from build123d import *

# Parameters (mm, degrees)
SKETCH1_W           = 64.8
SKETCH1_H           = 159
SKETCH1_R           = 1.5
BOSS_EXTRUDE1_DEPTH = 3
SKETCH7_W           = 2.2
SKETCH7_H           = 52
CUT_EXTRUDE4_DEPTH  = 86.901164136
CUT_EXTRUDE6_DEPTH  = 86.901164136
SKETCH12_R          = 1.25
CUT_EXTRUDE8_DEPTH  = 10


with BuildPart() as part:
    # Sketch1 → Boss-Extrude1 (new body)
    with BuildSketch(Plane(origin=(0, 0, 0), x_dir=(1, 0, 0), z_dir=(0, 1, 0))):
        Rectangle(SKETCH1_W, SKETCH1_H)
        with Locations(Location((-27.4, 69.5, 0), (0, 0, 270))):
            Circle(SKETCH1_R, mode=Mode.SUBTRACT)
        with Locations(Location((27.4, 69.5, 0), (0, 0, 270))):
            Circle(SKETCH1_R, mode=Mode.SUBTRACT)
        with Locations(Location((27.4, 31.5, 0), (0, 0, 270))):
            Circle(SKETCH1_R, mode=Mode.SUBTRACT)
        with Locations(Location((-27.4, 31.5, 0), (0, 0, 270))):
            Circle(SKETCH1_R, mode=Mode.SUBTRACT)
    extrude(amount=BOSS_EXTRUDE1_DEPTH)

    # Sketch7 → Cut-Extrude4 (cut, through all)
    with BuildSketch(Plane(origin=(0, 3, 0), x_dir=(1, 0, 0), z_dir=(0, 1, 0))):
        with Locations((-27.6, -8.5)):
            Rectangle(SKETCH7_W, SKETCH7_H)
        with Locations((27.6, -8.5)):
            Rectangle(SKETCH7_W, SKETCH7_H)
        with Locations((-21.9, -8.5)):
            Rectangle(SKETCH7_W, SKETCH7_H)
        with Locations((21.9, -8.5)):
            Rectangle(SKETCH7_W, SKETCH7_H)
    extrude(amount=-CUT_EXTRUDE4_DEPTH, mode=Mode.SUBTRACT)

    # Sketch9 → Cut-Extrude6 (cut, through all)
    with BuildSketch(Plane(origin=(0, 3, 0), x_dir=(1, 0, 0), z_dir=(0, 1, 0))):
        Polygon((-27.4, -65.75), (27.4, -65.75), (27.4, -58.25), (8.75, -58.25), (8.75, -50.25), (-8.75, -50.25), (-8.75, -58.25), (-27.4, -58.25), align=None)
    extrude(amount=-CUT_EXTRUDE6_DEPTH, mode=Mode.SUBTRACT)

    # Sketch12 → Cut-Extrude8 (cut)
    with BuildSketch(Plane(origin=(0, 3, 0), x_dir=(1, 0, 0), z_dir=(0, 1, 0))):
        with Locations(Location((-24.5, -47.5, 0), (0, 0, 270))):
            Circle(SKETCH12_R)
        with Locations(Location((24.5, -47.5, 0), (0, 0, 270))):
            Circle(SKETCH12_R)
        with Locations(Location((24.5, -76.5, 0), (0, 0, 270))):
            Circle(SKETCH12_R)
        with Locations(Location((-24.5, -76.5, 0), (0, 0, 270))):
            Circle(SKETCH12_R)
    extrude(amount=-CUT_EXTRUDE8_DEPTH, mode=Mode.SUBTRACT)


solid = part.part
Work out the finished part from the listing and answer in its coordinate system (mm). A direction names the side the tool comes from. Give positions to 0.01 mm unless a question says otherwise; leave off trailing zeros. Order: outer loops, then holes, each group sorted by start corner. A loop starts at its lowest first (then second) coordinate and runs counter-clockwise, first axis right, second up. Notation, with made-up numbers: M 4.25,-10 L 41.25,-10 A36 ccw 41.25,28 Z; hole C -8,83 d6. An arc over 180 degrees is marked long. Return JSON: item names as keys, results as strings.
Q1. Find section C-C, the plane z = 63. Write down the section's boundary in (x, y).
Answer below:
{"outline": "M -32.4,0 L -27.4,0 L -27.4,3 L -32.4,3 Z; M 27.4,0 L 32.4,0 L 32.4,3 L 27.4,3 Z"}
Q2. Find section B-B, the plane x = -12. Write down the section's boundary in (y, z).
Answer below:
{"outline": "M 0,-79.5 L 3,-79.5 L 3,58.25 L 0,58.25 Z; M 0,65.75 L 3,65.75 L 3,79.5 L 0,79.5 Z"}
Q3. Find the intervals of material crossed by line 1 along X through (y, z) = (2.3, 76.5); line 2 along X through (y, z) = (1.7, -31.5); line 3 along Z through (x, y) = (-22, 1.35), in increasing order. Write a range as [from, to].
Answer below:
{"line 1": "x = [-32.4, -25.75], [-23.25, 23.25], [25.75, 32.4]", "line 2": "x = [-32.4, -28.9], [-25.9, 25.9], [28.9, 32.4]", "line 3": "z = [-79.5, -17.5], [34.5, 58.25], [65.75, 79.5]"}
Q4. The mould has two halves that part along X. Classify faces 1 (the face through (-18, 2, 58.25)), 2 (the face through (-32.4, 1, 1)), 3 (the face through (0, 0, -1)): pulls with the +X half, pulls with the -X half, needs draft (parallel to the pull), parting line crosses it, or undercut.
Answer below:
{"face 1": "undercut", "face 2": "pulls with the -X half", "face 3": "needs draft"}
Q5. Find section A-A, the plane z = 18. Write down the section's boundary in (x, y), and give its area (3 significant figures).
Answer below:
{"outline": "M -32.4,0 L -28.7,0 L -28.7,3 L -32.4,3 Z; M -26.5,0 L -23,0 L -23,3 L -26.5,3 Z; M -20.8,0 L 20.8,0 L 20.8,3 L -20.8,3 Z; M 23,0 L 26.5,0 L 26.5,3 L 23,3 Z; M 28.7,0 L 32.4,0 L 32.4,3 L 28.7,3 Z", "area": "168 mm^2"}
Q6. Which of the six approach directions +Z, -Z, +X, -X, +Y, -Y give full straight-line access (tool end or side, diameter ignored) to faces 4 (the face through (0, 3, -1)), 5 (the face through (-27.4, 2, 62))?
Answer below:
{"face 4": "+Z, -Z, +X, -X, +Y", "face 5": "+Y, -Y"}
Q7. Find section D-D, the plane z = -31.5. Write down the section's boundary in (x, y), and give its area (3 significant figures).
Answer below:
{"outline": "M -32.4,0 L -28.9,0 L -28.9,3 L -32.4,3 Z; M -25.9,0 L 25.9,0 L 25.9,3 L -25.9,3 Z; M 28.9,0 L 32.4,0 L 32.4,3 L 28.9,3 Z", "area": "176 mm^2"}
Q8. This flat-tipped pin is pushed along its axis until it touches: pin 1 (2 mm diameter, centred on x = -24.5, z = 47.5, fed in from -Y). Where does it stop, or does it pass through?
Answer below:
{"pin 1": "passes through"}
